Part model, mm, in its own coordinate system. Round coordinates to 2 decimals unless told otherwise and drop trailing zeros. Answer as a JSON object with one key per item and string values.
```python
from build123d import *

# Parameters (mm, degrees)
CROQUIS11_R = 11
VACIADO5_T  = -4
REDONDEO3_R = 1


with BuildPart() as part:
    # Barrer4: sweep along a path in Croquis10
    with BuildLine(Plane(origin=(0, 0, 0), x_dir=(0, 0, -1), z_dir=(-1, 0, 0))) as barrer4_path:
        Line((0, 0), (0, -24.910858202))
        ThreePointArc((0, -24.910858202), (-13.332739449, -74.170158996), (-49.690658823, -109.979967076))
        ThreePointArc((-49.690658823, -109.979967076), (-107.587992383, -145.259844558), (-162.97033395, -184.369526621))
        ThreePointArc((-162.97033395, -184.369526621), (-210.828414492, -226.710036816), (-251.758207116, -275.780055692))
        ThreePointArc((-251.758207116, -275.780055692), (-295.61896572, -356.963847424), (-318.172480576, -446.439615948))
    # Croquis11 → Barrer4 (sweep)
    with BuildSketch(Plane(origin=(0, 0, 0), x_dir=(-1, 0, 0), z_dir=(0, 1, 0))):
        Circle(CROQUIS11_R)
    sweep(path=barrer4_path.line)

    # Vaciado5
    vaciado5_openings = [part.faces().sort_by_distance(p)[0] for p in [
        (0, 446.439615948, 318.172480576),
        (0, 0, 0),
    ]]
    offset(amount=VACIADO5_T, openings=vaciado5_openings, kind=Kind.INTERSECTION)

    # Redondeo3
    redondeo3_edges = [part.edges().sort_by_distance(p)[0] for p in [
        (11, 0, 0),
        (11, 446.439615948, 318.172480576),
    ]]
    fillet(redondeo3_edges, radius=REDONDEO3_R)


solid = part.part
```
Item 1: Drop flat-ended pins along their axis: P1, Ø1.5, axis at x = 1.5, y = 160, coming from the -Z side; P2, Ø5, axis at x = -6.5, z = 198.5, coming from the -Y side; P3, Ø5, axis at x = 6, z = 125, coming from the +Y side. Give the stop position or say it passes through.
Taken from the geometry:
{"P1": "z = 108.95", "P2": "y = 199.35", "P3": "y = 170.56"}
Item 2: Probe L1, parallel to Z at x = 0, y = 16.5; L2, parallel to Y at x = -0.5, z = 195.5; L3, parallel to X at y = 320, z = 275. List the from-to ranges inside material, lowest first. Write a range as from..to.
Taken from the geometry:
{"L1": "-11..-7, 7..11", "L2": "196.86..202.24, 221.32..226.89", "L3": "-10.45..-6.11, 6.11..10.45"}
Item 3: Two-plate mould, pull along X, no slides. Class faces 1 (the cylindrical face through (2.38, 13.12, -10.74)), 2 (the cylindrical face through (-6.466, 12.63, -2.681)), 3 (the flat face through (6.714, 446.134, 320.654)): pulls with the +X half, pulls with the -X half, needs draft (parallel to the pull), parting line crosses it, or undercut.
Taken from the geometry:
{"face 1": "parting line crosses it", "face 2": "undercut", "face 3": "needs draft"}
